Source: CAD feature listing. Evaluate the final solid. Frame: model axes, mm. A direction names the side the tool comes from. Round coordinates to 2 decimals unless told otherwise and drop trailing zeros. Order: outer loops, then holes, each group sorted by start corner. A loop starts at its lowest first (then second) coordinate and runs counter-clockwise, first axis right, second up. Notation, with made-up numbers: (21.25, 55.25) - (69.25, 55.25) arc R27 cw to (69.25, 86.25) - close; hole circle Ø1 at (88, -6.5). An arc over 180 degrees is marked (long way). Use one line per item in the form item = value. Start each with the question number.
Q1. Pin query (flat end, axial travel): pin 1 Ø2.5 at (y, z) = (-10, 3) entering from -X; pin 2 Ø12 at (x, y) = (6.5, -4) entering from -Z; pin 3 Ø1.5 at (x, z) = (-6.5, 2.5) entering from -Y; pin 4 Ø1.5 at (x, z) = (-15, 2.5) entering from -Y (3 decimals). Return the tip coordinate at first contact, or that it passes through.
Q2. Cut plane C-C, the plane x = -1. Return the cut outline in (y, z), and give its area (3 significant figures).
Q3. Ray query, line 1 (Y direction, x = -8, z = 0.7); line 2 (X direction, y = -10.5, z = 1.1) (3 decimals); line 3 (Y direction, x = -15.5, z = 0.75) (3 decimals). Return the intervals inside material, ascending. Write a range as [from, to].
Q4. Cut plane A-A, the plane z = 3.9. Return the cut outline in (x, y) (3 decimals).
Q5. Cut plane B-B, the plane y = 5. Return the cut outline in (x, z) (3 decimals), and give its area (3 significant figures).
Q6. Set-up query: faces 1 (the flat face through (-16, 3.175, 3)), 2 (the flat face through (3.81, -9, 3)), 3 (the flat face through (9, 11.43, 3)). Return all of +Z, -Z, +X, -X, +Y, -Y with unobstructed straight access to the full face (end or side cutting, diameter ignored); none if empty.
from build123d import *

# Parameters (mm, degrees)
SKETCH1_W           = 5.08
SKETCH1_H           = 6.35
SKETCH1_W_2         = 26.67
SKETCH1_H_2         = 12.7
SKETCH1_W_3         = 9.525
SKETCH1_H_3         = 5.08
BOSS_EXTRUDE1_DEPTH = 5.08


with BuildPart() as part:
    # Sketch1 → Boss-Extrude1 (new body)
    with BuildSketch(Plane.XY):
        with Locations((-15.875, 0)):
            Rectangle(SKETCH1_W, SKETCH1_H)
        Rectangle(SKETCH1_W_2, SKETCH1_H_2)
        with Locations((8.5725, 8.89)):
            Rectangle(SKETCH1_W_3, SKETCH1_H_3)
        with Locations((8.5725, -8.89)):
            Rectangle(SKETCH1_W_3, SKETCH1_H_3)
    extrude(amount=BOSS_EXTRUDE1_DEPTH)


solid = part.part
Completed:
q1.pin_1 = 3.81
q1.pin_2 = 0
q1.pin_3 = -6.35
q1.pin_4 = -3.175
q2.outline = (-6.35, 0) - (6.35, 0) - (6.35, 5.08) - (-6.35, 5.08) - close
q2.area = 64.5 mm2
q3.line_1 = [-6.35, 6.35]
q3.line_2 = [3.81, 13.335]
q3.line_3 = [-3.175, 3.175]
q4.outline = (-18.415, -3.175) - (-13.335, -3.175) - (-13.335, -6.35) - (3.81, -6.35) - (3.81, -11.43) - (13.335, -11.43) - (13.335, 11.43) - (3.81, 11.43) - (3.81, 6.35) - (-13.335, 6.35) - (-13.335, 3.175) - (-18.415, 3.175) - close
q5.outline = (-13.335, 0) - (13.335, 0) - (13.335, 5.08) - (-13.335, 5.08) - close
q5.area = 135 mm2
q6.face_1 = +Z, -Z, -X, +Y
q6.face_2 = +Z, -Z, -X, -Y
q6.face_3 = +Z, -Z, +X, -X, +Y
